Here's how the part is built. I have some questions about the finished solid (model axes, mm). A direction names the side the tool comes from. Round coordinates to 2 decimals unless told otherwise and drop trailing zeros. Write each loop counter-clockwise with the first axis right and the second up, starting at its lowest first coordinate (ties: lowest second). Pieces come first, ordered by that corner, then holes. Notation, with made-up numbers: M -31,-23 L 4,-23 A8 ccw 4,-9 Z; hole C 35,46 d6. An arc over 180 degrees is marked long. Use one line per item in the form item = value. Start each with the question number.
Q1. I want a section at B-B on z = 163.5. List the corners of the cut face in (x, y) for me.
Q2. I want a section at A-A on y = 10. List the corners of the cut face in (x, z) for me, and give its area (3 significant figures).
Q3. For faces 5 (the face through (0, 13, 275)), 6 (the face through (23.812, 13, 275)), which set-ups out of +Z, -Z, +X, -X, +Y, -Y let a thin tool reach every point of the face, with its end or its side?
Q4. We'd pull the mould along Y, two halves only. Please class faces 1 (the face through (13, 0, 275)), 2 (the face through (13, 23.812, 275)), 3 (the face through (13, 25.4, 275)), 4 (the face through (1, 13, 0)): +Y half, -Y half, draft (parallel to the pull), parting line (faces both ways), or undercut.
Q5. I need wall thicknesses on line 1 along Z through (x, y) = (12.7, 24.2) (3 decimals); line 2 along X through (y, z) = (9.5, 183). Which ranges of each line are inside material? Lowest first, please. Write a range as from..to.
Autodesk Inventor part; units mm, degrees
ref_plane "YZ Plane" through (0, 0, 0) normal (1, 0, 0) x (0, 1, 0)
ref_plane "XZ Plane" through (0, 0, 0) normal (0, 1, 0) x (-1, 0, 0)
ref_plane "XY Plane" through (0, 0, 0) normal (0, 0, 1) x (1, 0, 0)
sketch "Sketch1" plane through (0, 0, 0) normal (0, 0, 1) x (1, 0, 0)
  line L0 (0, 0) -> (25.4, 0)
  line L1 (25.4, 0) -> (25.4, 25.4)
  line L2 (25.4, 25.4) -> (0, 25.4)
  line L3 (0, 25.4) -> (0, 0)
  line L4 (1.5875, 1.5875) -> (23.8125, 1.5875)
  line L5 (23.8125, 1.5875) -> (23.8125, 23.8125)
  line L6 (23.8125, 23.8125) -> (1.5875, 23.8125)
  line L7 (1.5875, 23.8125) -> (1.5875, 1.5875)
  dimension "d0" = 25.4
  dimension "d1" = 25.4
  dimension "d2" = 1.5875
extrude "Extrusion1" add sketch "Sketch1" along normal blind 558.8
sketch "Sketch3" plane through (0, 25.4, 0) normal (0, 1, 0) x (1, 0, 0)
  line L0 (25.4, 0) -> (0, 0)
  line L1 (0, 0) -> (0, -558.8)
  line L2 (25.4, -558.8) -> (0, -558.8)
  line L3 (25.4, 0) -> (25.4, -558.8)
  point P0 (0, 0)
  point P1 (12.7, -279.4)
  dimension "d15" = 279.4
  dimension "d16" = 558.8
  dimension "d17" = 12.7
hole "Hole2" at (12.7, 25.4, 279.4) direction (0, -1, 0) diameter 6.35 end through all
sketch "Sketch4" plane through (0, 25.4, 0) normal (0, 1, 0) x (1, 0, 0)
  circle A0 centre (12.7, -279.4) radius 3.175
  line L0 (25.4, 0) -> (0, 0)
  line L1 (0, 0) -> (0, -558.8)
  line L2 (25.4, -558.8) -> (0, -558.8)
  line L3 (25.4, 0) -> (25.4, -558.8)
  point P0 (0, 0)
  point P1 (12.7, -546.1)
  dimension "d25" = 12.7
  dimension "d26" = 12.7
  dimension "d27" = 12.7
hole "Hole3" at (12.7, 25.4, 546.1) direction (0, -1, 0) diameter 6.35 end through all
properties part number "ScissorLiftBarBottom" material "Aluminum 6061"
Reported:
q1.outline = M 0,0 L 25.4,0 L 25.4,25.4 L 0,25.4 Z; hole M 1.59,1.59 L 23.81,1.59 L 23.81,23.81 L 1.59,23.81 Z
q2.outline = M 0,0 L 1.59,0 L 1.59,558.8 L 0,558.8 Z; M 23.81,0 L 25.4,0 L 25.4,558.8 L 23.81,558.8 Z
q2.area = 1,770 mm^2
q3.face_5 = +Z, -Z, -X, +Y, -Y
q3.face_6 = +Z, -Z
q4.face_1 = -Y half
q4.face_2 = undercut
q4.face_3 = +Y half
q4.face_4 = draft
q5.line_1 = 0..276.225, 282.575..542.925, 549.275..558.8
q5.line_2 = 0..1.59, 23.81..25.4
